Geometry check sheet. Reference: the model listing, model coordinates, mm. Face numbers are marked on the shaded views. Give positions to 0.01 mm unless a question says otherwise; leave off trailing zeros. Loops run counter-clockwise (first coordinate to the right, second up) from the corner with the lowest first, then second, coordinate; pieces in that order, holes last. Notation, with made-up numbers: (44.5, 7.25) -> (92.5, 7.25) arc R20 ccw to (92.5, 26.25) -> close; hole circle Ø9 at (36.25, 13). An arc over 180 degrees is marked (long way). Write item = value, one per line.
```python
from build123d import *

# Parameters (mm, degrees)
SKETCH1_R           = 74.93
SKETCH1_R_2         = 3.175
BOSS_EXTRUDE1_DEPTH = 4.1275
SKETCH2_R           = 73.66
CUT_EXTRUDE1_DEPTH  = 2.8575


with BuildPart() as part:
    # Sketch1 → Boss-Extrude1 (new body)
    with BuildSketch(Plane.XY):
        Circle(SKETCH1_R)
        Circle(SKETCH1_R_2, mode=Mode.SUBTRACT)
    extrude(amount=BOSS_EXTRUDE1_DEPTH)

    # Sketch2 → Cut-Extrude1 (cut)
    with BuildSketch(Plane(origin=(0, 0, 0), x_dir=(-1, 0, 0), z_dir=(0, 0, -1))):
        Circle(SKETCH2_R)
    extrude(amount=-CUT_EXTRUDE1_DEPTH, mode=Mode.SUBTRACT)

    # Sketch3 → Revolve1 (revolve)
    with BuildSketch(Plane(origin=(0, 0, 0), x_dir=(0, 0, -1), z_dir=(1, 0, 0)), mode=Mode.PRIVATE) as revolve1_sk:
        Polygon((-5.6515, 68.400374819), (-4.1275, 69.162374819), (-4.1275, 68.400374819), align=None)
    revolve(revolve1_sk.sketch.rotate(Axis((0, 68.400374819, 5.6515), (0, 0, -1)), 270), axis=Axis((0, 68.400374819, 5.6515), (0, 0, -1)))


solid = part.part
```
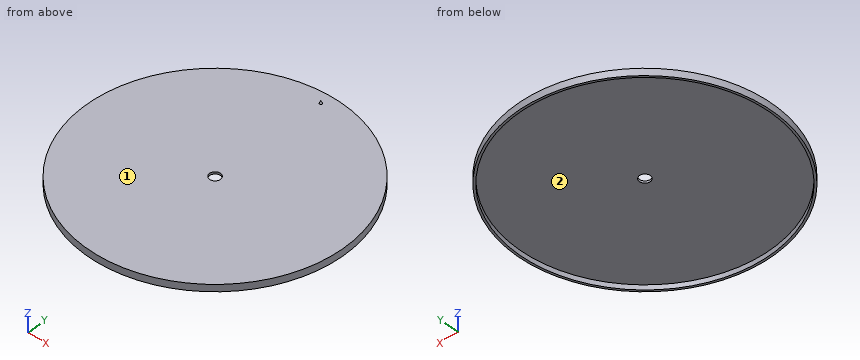
Item 1: Thickness scan on L1, parallel to Y at x = 0, z = 3.2 (3 decimals); L2, parallel to Y at x = 0, z = 1.95; L3, parallel to Z at x = -18, y = 12. Record the ranges inside material, lowest first. Write a range as [from, to].
Answer:
L1 = [-74.93, -3.175], [3.175, 74.93]
L2 = [-74.93, -73.66], [73.66, 74.93]
L3 = [2.86, 4.13]
Item 2: Section check A-A, the plane y = 0. Record the cut outline in (x, z) (1 decimal), plus the area to 3 significant figures.
Answer:
outline = (-74.9, 0) -> (-73.7, 0) -> (-73.7, 2.9) -> (-3.2, 2.9) -> (-3.2, 4.1) -> (-74.9, 4.1) -> close; (3.2, 2.9) -> (73.7, 2.9) -> (73.7, 0) -> (74.9, 0) -> (74.9, 4.1) -> (3.2, 4.1) -> close
area = 190 mm^2
Item 3: Section check C-C, the plane y = -41.5. Record the cut outline in (x, z), plus the area to 3 significant figures.
Answer:
outline = (-62.39, 0) -> (-60.86, 0) -> (-60.86, 2.86) -> (60.86, 2.86) -> (60.86, 0) -> (62.39, 0) -> (62.39, 4.13) -> (-62.39, 4.13) -> close
area = 167 mm^2
Item 4: Section check B-B, the plane z = 1.75. Record the cut outline in (x, y).
Answer:
outline = circle Ø149.86 at (0, 0); hole circle Ø147.32 at (0, 0)
Item 5: Section check D-D, the plane x = 7.5. Record the cut outline in (y, z).
Answer:
outline = (-74.55, 0) -> (-73.28, 0) -> (-73.28, 2.86) -> (73.28, 2.86) -> (73.28, 0) -> (74.55, 0) -> (74.55, 4.13) -> (-74.55, 4.13) -> close
Item 6: Gauge pin test, flat ends, axial feed: pin 1 (3 mm diameter, centred on x = -27, z = 3, fed in from +Y); pin 2 (8 mm diameter, centred on x = -10.5, y = -18, fed in from -Z); pin 3 (10 mm diameter, centred on x = 0, y = 0, fed in from +Z). Record the tip position at first contact, or that the pin passes through.
Answer:
pin_1 = 70.46
pin_2 = 2.86
pin_3 = 4.13
Item 7: Draft check along X on the marked faces 1 and 2. Enter one of: +X half, -X half, draft (parallel to the pull), parting line (faces both ways), or undercut.
Answer:
face_1 = draft
face_2 = undercut
